Can you work these out from the model? Positions are in its coordinate system, mm. A direction names the side the tool comes from. Coordinates: 2 decimals unless noted, no trailing zeros. Order: outer loops, then holes, each group sorted by start corner. A loop starts at its lowest first (then second) coordinate and runs counter-clockwise, first axis right, second up. Notation, with made-up numbers: (-14, 69) -> (3, 69) arc R4 cw to (3, 76) -> close; hole circle Ø5 at (13.25, 22). An arc over 180 degrees is marked (long way). Return JSON: item names as keys, results as strings. Group by question number.
1) For faces 1 (the flat face through (0, 8.5, 3)), 2 (the flat face through (-22, 0, 11)), 3 (the flat face through (25, -6, 7)), 4 (the flat face through (-12.54, 6.98, 11.55)), 5 (the flat face through (23, 0, 18)), which set-ups out of +Z, -Z, +X, -X, +Y, -Y let a thin tool reach every point of the face, with its end or its side?
2) If we section it at B-B, the plane y = 0: State how many separate pieces and enclosed holes the cut face has, then the cut area to 3 significant figures.
3) If we section it at A-A, the plane x = -11: Please give me the cut outline in (y, z).
4) If we section it at D-D, the plane x = -4.5: Please give me the cut outline in (y, z).
5) Thinking about a two-plate mould opening in Z: for faces 6 (the cylindrical face through (-25.5, -0.9, 7.8)), 7 (the flat face through (0, 0, 0)), 8 (the flat face through (22, 0, 11)), which applies, +Z half, -Z half, draft (parallel to the pull), parting line (faces both ways), or undercut?
6) For pin 1 (5 mm diameter, centred on y = -3.5, z = 2.5, fed in from +X); pin 2 (6 mm diameter, centred on x = -12, y = 0, fed in from +Z); pin 3 (1.5 mm diameter, centred on y = 5, z = 16, fed in from -X), each with a flat end and sliding along its axis, tell me the tip position at first contact or that it passes through.
7) If I drill on probe 1 along Y at (x, z) = (-18.5, 14.5); probe 2 along Y at (x, z) = (12, 2.15); probe 3 along Z at (x, y) = (23.4, 0), over which ranges is the centre line in solid material (lowest first)? Write a range as from..to.
from build123d import *
from OCP.BRepFilletAPI import BRepFilletAPI_MakeChamfer

# Parameters (mm, degrees)
SKETCH_1_W               = 50
SKETCH_1_H               = 17
EXTRUDE_1_DEPTH          = 18
SKETCH_2_W               = 44
SKETCH_2_H               = 11
CUT_EXTRUDE_1_DEPTH      = 15
CUT_EXTRUDE_2_DEPTH      = 36.185224172
CUT_EXTRUDE_2_DEPTH_BACK = 17
SKETCH_4_R               = 2.6
CUT_EXTRUDE_4_DEPTH      = 3
SKETCH_5_R               = 4
SKETCH_5_R_2             = 1.5
EXTRUDE_2_DEPTH          = 4
EXTRUDE_START            = 4
SKETCH_6_R               = 4
SKETCH_6_R_2             = 1.5
EXTRUDE_3_DEPTH          = 4
CHAMFER_1_SIZE           = 2
CHAMFER_1_SIZE_2         = 4
CUT_EXTRUDE_START        = -50
SKETCH_7_R               = 1.5
CUT_EXTRUDE_5_DEPTH      = 50


with BuildPart() as part:
    # 草图1 → 凸台-拉伸1 (new body)
    with BuildSketch(Plane.XY):
        Rectangle(SKETCH_1_W, SKETCH_1_H)
    extrude(amount=EXTRUDE_1_DEPTH)

    # 草图2 → 切除-拉伸1 (cut)
    with BuildSketch(Plane.XY.offset(18)):
        Rectangle(SKETCH_2_W, SKETCH_2_H)
    extrude(amount=-CUT_EXTRUDE_1_DEPTH, mode=Mode.SUBTRACT)

    # 草图3 → 切除-拉伸2 (cut, two sides: drawn at the far end of the back side and taken through both)
    with BuildSketch(Plane(origin=(0, 8.5, 0), x_dir=(1, 0, 0), z_dir=(0, 1, 0)).offset(-CUT_EXTRUDE_2_DEPTH_BACK)):
        with BuildLine():
            Line((-113.428530012, -80.337634099), (-22, -18))
            Line((-22, -18), (-2.816684123, -4.920466448))
            ThreePointArc((-2.816684123, -4.920466448), (0, -4.051603162), (2.816684123, -4.920466448))
            Line((2.816684123, -4.920466448), (22, -18))
            Line((22, -18), (113.428530012, -80.337634099))
            Line((113.428530012, -80.337634099), (113.428530012, -301.653306613))
            Line((113.428530012, -301.653306613), (-113.428530012, -301.653306613))
            Line((-113.428530012, -301.653306613), (-113.428530012, -80.337634099))
        make_face()
    extrude(amount=CUT_EXTRUDE_2_DEPTH + CUT_EXTRUDE_2_DEPTH_BACK, mode=Mode.SUBTRACT)

    # 草图4 → 切除-拉伸4 (cut)
    with BuildSketch(Plane.XY.offset(3)):
        with Locations((-12, 0)):
            Circle(SKETCH_4_R)
        with Locations(Location((12, 0, 0), (0, 0, 180))):
            Circle(SKETCH_4_R)
    extrude(amount=-CUT_EXTRUDE_4_DEPTH, mode=Mode.SUBTRACT)

    # 草图5 → 凸台-拉伸2 (add)
    with BuildSketch(Plane.ZY.offset(25)):
        with Locations(Location((9, 0, 0), (0, 0, 180))):
            Circle(SKETCH_5_R)
        with Locations((9, 0)):
            Circle(SKETCH_5_R_2, mode=Mode.SUBTRACT)
    extrude(amount=EXTRUDE_2_DEPTH)

    # 草图6 → 凸台-拉伸3 (add)
    with BuildSketch(Plane(origin=(25, 0, 0), x_dir=(0, 0, -1), z_dir=(1, 0, 0)).offset(EXTRUDE_START)):
        with Locations((-9, 0)):
            Circle(SKETCH_6_R)
        with Locations(Location((-9, 0, 0), (0, 0, 180))):
            Circle(SKETCH_6_R_2, mode=Mode.SUBTRACT)
    extrude(amount=-EXTRUDE_3_DEPTH)

    # 倒角1
    chamfer_1_edges_1 = [part.edges().sort_by_distance(p)[0] for p in [
        (-25, 0, 13),
    ]]
    chamfer_1_side_1 = [part.faces().sort_by_distance(p)[0] for p in [
        (-25, 0, 13.04),
    ]]
    chamfer_1_edges_2 = [part.edges().sort_by_distance(p)[0] for p in [
        (25, 0, 13),
    ]]
    chamfer_1_side_2 = [part.faces().sort_by_distance(p)[0] for p in [
        (25, 0, 13.04),
    ]]
    chamfer_1 = BRepFilletAPI_MakeChamfer(part.part.solid().wrapped)
    for e in chamfer_1_edges_1:
        chamfer_1.Add(CHAMFER_1_SIZE - 0.0001, CHAMFER_1_SIZE_2 - 0.0001, e.wrapped, chamfer_1_side_1[0].wrapped)
    for e in chamfer_1_edges_2:
        chamfer_1.Add(CHAMFER_1_SIZE - 0.0001, CHAMFER_1_SIZE_2 - 0.0001, e.wrapped, chamfer_1_side_2[0].wrapped)
    add(Compound.cast(chamfer_1.Shape()), mode=Mode.REPLACE)  # a hair under: the kernel refuses the full size

    # 草图7 → 切除-拉伸5 (cut)
    with BuildSketch(Plane.ZY.offset(25).offset(CUT_EXTRUDE_START)):
        with Locations((9, 0)):
            Circle(SKETCH_7_R)
    extrude(amount=CUT_EXTRUDE_5_DEPTH, mode=Mode.SUBTRACT)


solid = part.part
Result sheet:
{
 "1": {"face 1": "+Z, -Z, +X, -X, +Y", "face 2": "+Z", "face 3": "+X", "face 4": "+Z, +Y, -Y", "face 5": "+Z, +X, -X, +Y, -Y"},
 "2": {"separate pieces": "5", "enclosed holes": "0", "area": "247 mm2"},
 "3": {"outline": "(-8.5, 0) -> (-2.4, 0) -> (-2.4, 3) -> (-5.5, 3) -> (-5.5, 10.5) -> (-8.5, 10.5) -> close; (2.4, 0) -> (8.5, 0) -> (8.5, 10.5) -> (5.5, 10.5) -> (5.5, 3) -> (2.4, 3) -> close"},
 "4": {"outline": "(-8.5, 0) -> (8.5, 0) -> (8.5, 6.07) -> (5.5, 6.07) -> (5.5, 3) -> (-5.5, 3) -> (-5.5, 6.07) -> (-8.5, 6.07) -> close"},
 "5": {"face 6": "undercut", "face 7": "-Z half", "face 8": "draft"},
 "6": {"pin 1": "stops at x = 27.24", "pin 2": "stops at z = 3", "pin 3": "stops at x = -25"},
 "7": {"probe 1": "y = -8.5..-5.5, 5.5..8.5", "probe 2": "y = -8.5..-2.6, 2.6..8.5", "probe 3": "z = 0..7.5, 10.5..18"}
}
